For this review, take the finished solid that the model builds, in its own axes (mm). Round coordinates to 2 decimals unless told otherwise and drop trailing zeros. Write each loop counter-clockwise with the first axis right and the second up, starting at its lowest first coordinate (ties: lowest second). Pieces come first, ordered by that corner, then holes. Notation, with made-up numbers: (-2.75, 27.25) - (56.25, 27.25) arc R21 cw to (56.25, 50.25) - close; hole circle Ø7 at (-25.75, -16.75). An arc over 180 degrees is marked (long way). One line per item, written item: value. Start each with the question number.
Q1. Clearance check with a flat-ended pin moving along its axis: pin 1 Ø1 at (y, z) = (2.5, 1.5) entering from -X. State where the tip first meets the part, or that it passes through.
Q2. Add section A-A on y = 1.75. Write out the cut boundary in (x, z), and give its area (3 significant figures).
Q3. For probe 1 along X at (y, z) = (0.3, -0.1); probe 2 along Z at (x, y) = (6.5, 1.15); probe 3 along X at (y, z) = (1.6, -0.55), list the stretches that pass through material, from the lowest coordinate up.
```python
from build123d import *

# Parameters (mm, degrees)
BOSS_EXTRU_1_DEPTH = 4
CHANFREIN1_SIZE    = 0.1


with BuildPart() as part:
    # Esquisse1 → Boss.-Extru.1 (new body)
    with BuildSketch(Plane(origin=(0, 0, 0), x_dir=(1, 0, 0), z_dir=(0, 1, 0))):
        with BuildLine():
            Line((-5.5, 2), (5.5, 2))
            ThreePointArc((5.5, 2), (7.5, 0), (5.5, -2))
            Line((5.5, -2), (-5.5, -2))
            ThreePointArc((-5.5, -2), (-7.5, 0), (-5.5, 2))
        make_face()
    extrude(amount=BOSS_EXTRU_1_DEPTH)

    # Chanfrein1
    chanfrein1_edges = [part.edges().sort_by_distance(p)[0] for p in [
        (7.5, 4, 0),
        (0, 4, -2),
        (-7.5, 4, 0),
        (0, 0, -2),
        (7.5, 0, 0),
        (0, 0, 2),
        (-7.5, 0, 0),
        (0, 4, 2),
    ]]
    chamfer(chanfrein1_edges, length=CHANFREIN1_SIZE)


solid = part.part
```
Result set:
1. pin 1: stops at x = -7.23
2. outline: (-5.5, -2) - (5.5, -2) arc R2 ccw to (5.5, 2) - (-5.5, 2) arc R2 ccw to start
2. area: 56.6 mm^2
3. probe 1: x = -7.5 to 7.5
3. probe 2: z = -1.73 to 1.73
3. probe 3: x = -7.42 to 7.42
